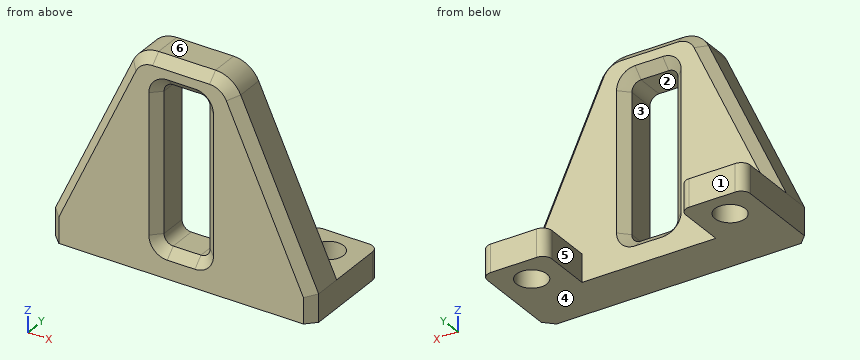
```python
from build123d import *

# Parameters (mm, degrees)
SKETCH_1_R          = 1.65
EXTRUDE_1_DEPTH     = 3
EXTRUDE_2_DEPTH     = 5
SKETCH_3_W          = 5
SKETCH_3_H          = 17
CUT_EXTRUDE_1_DEPTH = 12
FILLET_1_R          = 3
FILLET_2_R          = 1
CHAMFER_1_SIZE      = 1
FILLET_3_R          = 1
CHAMFER_2_SIZE      = 1


with BuildPart() as part:
    # ｽｹｯﾁ1 → ﾎﾞｽ - 押し出し1 (new body)
    with BuildSketch(Plane.XY):
        Polygon((-7.25, -3), (7.25, -3), (7.25, 3), (14.25, 3), (14.25, -8), (-14.25, -8), (-14.25, 3), (-7.25, 3), align=None)
        with Locations((10.75, 0)):
            Circle(SKETCH_1_R, mode=Mode.SUBTRACT)
        with Locations((-10.75, 0)):
            Circle(SKETCH_1_R, mode=Mode.SUBTRACT)
    extrude(amount=EXTRUDE_1_DEPTH)

    # ｽｹｯﾁ2 → ﾎﾞｽ - 押し出し2 (add)
    with BuildSketch(Plane.XZ.offset(8)):
        Polygon((-14.25, 3), (-5, 23), (5, 23), (14.25, 3), align=None)
    extrude(amount=-EXTRUDE_2_DEPTH)

    # ｽｹｯﾁ3 → ｶｯﾄ - 押し出し1 (cut, through all)
    with BuildSketch(Plane.XZ.offset(8)):
        with Locations((0, 11.5)):
            Rectangle(SKETCH_3_W, SKETCH_3_H)
    extrude(amount=-CUT_EXTRUDE_1_DEPTH, mode=Mode.SUBTRACT)

    # ﾌｨﾚｯﾄ1
    fillet_1_edges = [part.edges().sort_by_distance(p)[0] for p in [
        (-5, -5.5, 23),
        (5, -5.5, 23),
    ]]
    fillet(fillet_1_edges, radius=FILLET_1_R)

    # ﾌｨﾚｯﾄ2
    fillet_2_edges = [part.edges().sort_by_distance(p)[0] for p in [
        (7.25, 3, 1.5),
        (14.25, 3, 1.5),
        (-14.25, 3, 1.5),
        (-7.25, 3, 1.5),
    ]]
    fillet(fillet_2_edges, radius=FILLET_2_R)

    # 面取り1
    chamfer_1_edges = [part.edges().sort_by_distance(p)[0] for p in [
        (14.25, -8, 1.5),
        (-14.25, -8, 1.5),
        (10.027529355, -3, 12.12966626),
        (10.027529355, -8, 12.12966626),
        (0, -8, 23),
        (0, -3, 23),
        (-10.027529355, -8, 12.12966626),
        (4.69803687, -8, 22.527646886),
        (-4.69803687, -8, 22.527646886),
        (-10.027529355, -3, 12.12966626),
        (4.69803687, -3, 22.527646886),
        (-4.69803687, -3, 22.527646886),
    ]]
    chamfer(chamfer_1_edges, length=CHAMFER_1_SIZE)

    # ﾌｨﾚｯﾄ3
    fillet_3_edges = [part.edges().sort_by_distance(p)[0] for p in [
        (2.5, -5.5, 20),
        (2.5, -5.5, 3),
        (-2.5, -5.5, 3),
        (-2.5, -5.5, 20),
    ]]
    fillet(fillet_3_edges, radius=FILLET_3_R)

    # 面取り2
    chamfer_2_edges = [part.edges().sort_by_distance(p)[0] for p in [
        (2.5, -8, 11.5),
        (2.5, -3, 11.5),
        (0, -8, 3),
        (0, -3, 3),
        (-2.5, -8, 11.5),
        (-2.5, -3, 11.5),
        (0, -8, 20),
        (0, -3, 20),
        (2.207106781, -8, 3.292893219),
        (2.207106781, -3, 3.292893219),
        (-2.207106781, -8, 3.292893219),
        (-2.207106781, -3, 3.292893219),
        (2.207106781, -8, 19.707106781),
        (2.207106781, -3, 19.707106781),
        (-2.207106781, -8, 19.707106781),
        (-2.207106781, -3, 19.707106781),
    ]]
    chamfer(chamfer_2_edges, length=CHAMFER_2_SIZE)


solid = part.part
```
Part model, mm, in its own coordinate system. Face numbers are marked on the shaded views. A direction names the side the tool comes from. Round coordinates to 2 decimals unless told otherwise and drop trailing zeros. Order: outer loops, then holes, each group sorted by start corner. A loop starts at its lowest first (then second) coordinate and runs counter-clockwise, first axis right, second up. Notation, with made-up numbers: M -32,4.5 L -6,4.5 A14 cw -6,8.5 Z; hole C 74.25,-37 d9. An arc over 180 degrees is marked long. Answer in a Markdown table with one row per item. Add a question column.
Q1. Cut at A-A on y = -5.75. Give the cut face in (x, z).
Q2. Cut at C-C on y = 0. Give the cut face in (x, z).
Q3. Cut at D-D on z = 5. Give the cut face in (x, y) (3 decimals).
Q4. Wall check: L1, parallel to Y at x = 10.75, z = 2.1; L2, parallel to Z at x = -1.5, y = -5.5; L3, parallel to X at y = -6, z = 13.5. Give the ranges that are in metal, low to high. Write a range as from..to.
Q5. 3-axis set-ups, long thin cutter, end or side, ignore diameter. For the marked faces 1 and 2: which of +Z, -Z, +X, -X, +Y, -Y reach the whole face in a straight line?
Q6. Mould opens along Z. For the marked faces 3, 4, 5 and 6 say: +Z half, -Z half, draft (parallel to the pull), parting line (faces both ways), or undercut.
Q7. Pin check, flat tips, straight feed: pin 1 (11 mm diameter, centred on x = 5, z = 14.5, fed in from +Y); pin 2 (0.9 mm diameter, centred on y = -5, z = 13.5, fed in from -X); pin 3 (1.5 mm diameter, centred on y = -5, z = 14, fed in from +X). Stop position of each tip, or through.
Q8. Cut at B-B on x = 9.75. Give the cut face in (y, z), and give its area (3 significant figures).
Established:
| question | item | result |
|---|---|---|
| 1 | outline | M -14.25,0 L 14.25,0 L 14.25,3 L 5.81,21.26 A3 ccw 3.08,23 L -3.08,23 A3 ccw -5.81,21.26 L -14.25,3 Z; hole M -2.5,4 A1 ccw -1.5,3 L 1.5,3 A1 ccw 2.5,4 L 2.5,19 A1 ccw 1.5,20 L -1.5,20 A1 ccw -2.5,19 Z |
| 2 | outline | M -14.25,0 L -12.4,0 L -12.4,3 L -14.25,3 Z; M -9.1,0 L -7.25,0 L -7.25,3 L -9.1,3 Z; M 7.25,0 L 9.1,0 L 9.1,3 L 7.25,3 Z; M 12.4,0 L 14.25,0 L 14.25,3 L 12.4,3 Z |
| 3 | outline | M -13.325,-7 L -12.223,-8 L -3.5,-8 L -2.5,-7 L -2.5,-4 L -3.5,-3 L -12.223,-3 L -13.325,-4 Z; M 2.5,-7 L 3.5,-8 L 12.223,-8 L 13.325,-7 L 13.325,-4 L 12.223,-3 L 3.5,-3 L 2.5,-4 Z |
| 4 | L1 | y = -8..-1.65, 1.65..3 |
| 4 | L2 | z = 0..3, 20..23 |
| 4 | L3 | x = -9.39..-2.5, 2.5..9.39 |
| 5 | face 1 | +Z, -Z, +X, -X, +Y |
| 5 | face 2 | +Y, -Y |
| 6 | face 3 | undercut |
| 6 | face 4 | -Z half |
| 6 | face 5 | draft |
| 6 | face 6 | +Z half |
| 7 | pin 1 | stops at y = -3 |
| 7 | pin 2 | stops at x = -9.6 |
| 7 | pin 3 | stops at x = 9.51 |
| 8 | outline | M -8,0 L -1.31,0 L -1.31,3 L -3,3 L -3,10.35 L -4,12.73 L -7,12.73 L -8,10.35 Z; M 1.31,0 L 3,0 L 3,3 L 1.31,3 Z |
| 8 | area | 71.4 mm2 |
